```python
from build123d import *

# Parameters (mm, degrees)
ESQUISSE1_W             = 9.73
ESQUISSE1_H             = 5.03
BOSS_EXTRU_1_DEPTH      = 3.31
ESQUISSE3_W             = 3.841312789
ESQUISSE3_H             = 3.396529204
BOSS_EXTRU_2_DEPTH      = 0.1
BOSS_EXTRU_2_DEPTH_BACK = 1
ENL_V_MAT_EXTRU_1_DEPTH = 10.98001124
ESQUISSE5_W             = 5.874071128
ESQUISSE5_H             = 5.928896842
ENL_V_MAT_EXTRU_2_DEPTH = 2.1
ENL_V_MAT_EXTRU_4_DEPTH = 2.1
CONG_1_R                = 0.75
CONG_2_R                = 0.75


with BuildPart() as part:
    # Esquisse1 → Boss.-Extru.1 (new body)
    with BuildSketch(Plane.XY):
        Rectangle(ESQUISSE1_W, ESQUISSE1_H)
    extrude(amount=BOSS_EXTRU_1_DEPTH)

    # Esquisse3 → Boss.-Extru.2 (add, two sides)
    with BuildSketch(Plane(origin=(0, 0, 0), x_dir=(-1, 0, 0), z_dir=(0, 0, -1))) as boss_extru_2_sk:
        with Locations((-3.194354846, 0)):
            Rectangle(ESQUISSE3_W, ESQUISSE3_H)
        with Locations((3.194354846, 0)):
            Rectangle(ESQUISSE3_W, ESQUISSE3_H)
    extrude(amount=BOSS_EXTRU_2_DEPTH)
    extrude(boss_extru_2_sk.sketch, amount=-BOSS_EXTRU_2_DEPTH_BACK)

    # Esquisse4 → Enlèv. mat.-Extru.1 (cut, through all)
    with BuildSketch(Plane(origin=(4.865, 0, 0), x_dir=(0, 0, -1), z_dir=(1, 0, 0))):
        Polygon((-1.655, -2.515), (-3.31, -2.017151535), (-3.31, 2.017151535), (-1.655, 2.515), (-1.655, 2.602439027), (-3.426184741, 2.639019495), (-3.454926537, -2.688664416), (-1.655, -2.688664416), align=None)
    extrude(amount=-ENL_V_MAT_EXTRU_1_DEPTH, mode=Mode.SUBTRACT)

    # Esquisse5 → Enlèv. mat.-Extru.2 (cut)
    with BuildSketch(Plane.XY.offset(3.31)):
        with Locations((0, 0.049057066)):
            Rectangle(ESQUISSE5_W, ESQUISSE5_H)
    extrude(amount=-ENL_V_MAT_EXTRU_2_DEPTH, mode=Mode.SUBTRACT)

    # Esquisse6 → Enlèv. mat.-Extru.4 (cut)
    with BuildSketch(Plane.XY.offset(3.31)):
        Polygon((-2.937035564, 1.938709767), (-2.937035564, -1.938709767), (4.353991242, -1.938709767), (4.353991242, -0.833970123), (3.541647976, -0.833970123), (3.541647976, 0.833970123), (4.353991242, 0.833970123), (4.353991242, 1.938709767), align=None)
        Polygon((-4.353991242, -0.833970123), (-4.353991242, -1.938709767), (-2.937035564, -1.938709767), (-2.937035564, 1.938709767), (-4.353991242, 1.938709767), (-4.353991242, 0.833970123), (-3.541647976, 0.833970123), (-3.541647976, -0.833970123), align=None)
    extrude(amount=-ENL_V_MAT_EXTRU_4_DEPTH, mode=Mode.SUBTRACT)

    # Congé1
    cong_1_edges = [part.edges().sort_by_distance(p)[0] for p in [
        (-2.937035564, 2.226854883, 1.21),
        (2.937035564, 2.226854883, 1.21),
        (2.937035564, -2.226854883, 1.21),
        (-2.937035564, -2.226854883, 1.21),
    ]]
    fillet(cong_1_edges, radius=CONG_1_R)

    # Congé2
    cong_2_edges = [part.edges().sort_by_distance(p)[0] for p in [
        (2.937035564, 1.977930651, 3.31),
        (-2.937035564, -1.977930651, 3.31),
        (-2.937035564, 1.977930651, 3.31),
        (2.937035564, -1.977930651, 3.31),
    ]]
    fillet(cong_2_edges, radius=CONG_2_R)


solid = part.part
```
Geometry: final body of the model. Coordinates: model frame, mm. A direction names the side the tool comes from. Round coordinates to 2 decimals unless told otherwise and drop trailing zeros. Order: outer loops, then holes, each group sorted by start corner. A loop starts at its lowest first (then second) coordinate and runs counter-clockwise, first axis right, second up. Notation, with made-up numbers: (-2, -26) -> (8, -26) arc R10 cw to (8, -9) -> close; hole circle Ø11 at (3, 50). An arc over 180 degrees is marked (long way). Use CSV: the item, a comma, the result in double quotes. Start each with the question number.
1) Section D-D (z = 0.65). Return the cut outline in (x, y) (3 decimals), and give its area (3 significant figures).
2) First-contact query: pin 1 Ø1.5 at (x, z) = (4, 3) entering from +Y; pin 2 Ø3 at (x, y) = (-1.5, 0) entering from +Z; pin 3 Ø0.8 at (y, z) = (0, 2.5) entering from +X (3 decimals). Flat tips, straight axial feed; report the tip coordinate or a pass-through.
3) Set-up query: faces 1 (the face through (4, -0.834, 2)), 2 (the face through (3, 0, -0.1)). Return all of +Z, -Z, +X, -X, +Y, -Y with unobstructed straight access to the full face (end or side cutting, diameter ignored); none if empty.
4) Section A-A (z = 2.8). Return the cut outline in (x, y) (3 decimals), and give its area (3 significant figures).
5) Section C-C (y = -1.8). Return the cut outline in (x, z) (3 decimals), and give its area (3 significant figures).
6) Draft query along X for faces 3 (the face through (3.542, 0, 2)), 4 (the face through (5.115, 0, 0.4)), 5 (the face through (0, -2.515, 1)). Return one class per face: +X half, -X half, draft (parallel to the pull), parting line (faces both ways), or undercut.
7) Material intervals for line 1 along X through (y, z) = (-1.4, 2.55) (3 decimals); line 2 along X through (y, z) = (0.8, 3) (3 decimals); line 3 along Y through (x, z) = (4, 2.3), sorted ascending. Write a range as from..to.
8) Section B-B (x = 1.5). Return the cut outline in (y, z) (3 decimals).
Returned:
1,outline,"(-5.115, -1.698) -> (-4.865, -1.698) -> (-4.865, -2.515) -> (4.865, -2.515) -> (4.865, -1.698) -> (5.115, -1.698) -> (5.115, 1.698) -> (4.865, 1.698) -> (4.865, 2.515) -> (-4.865, 2.515) -> (-4.865, 1.698) -> (-5.115, 1.698) -> close"
1,area,"50.6 mm²"
2,pin 1,"stops at y = 2.34"
2,pin 2,"stops at z = 1.21"
2,pin 3,"stops at x = 4.865"
3,face 1,"+Z"
3,face 2,"-Z, +X, -X, +Y, -Y"
4,outline,"(-4.865, -2.171) -> (-2.976, -2.171) -> (-2.976, -1.939) -> (-4.354, -1.939) -> (-4.354, -0.834) -> (-3.542, -0.834) -> (-3.542, 0.834) -> (-4.354, 0.834) -> (-4.354, 1.939) -> (-2.976, 1.939) -> (-2.976, 2.171) -> (-4.865, 2.171) -> close; (2.976, -2.171) -> (4.865, -2.171) -> (4.865, 2.171) -> (2.976, 2.171) -> (2.976, 1.939) -> (4.354, 1.939) -> (4.354, 0.834) -> (3.542, 0.834) -> (3.542, -0.834) -> (4.354, -0.834) -> (4.354, -1.939) -> (2.976, -1.939) -> close"
4,area,"8.42 mm²"
5,outline,"(-4.865, 0) -> (4.865, 0) -> (4.865, 3.31) -> (4.354, 3.31) -> (4.354, 1.21) -> (-4.354, 1.21) -> (-4.354, 3.31) -> (-4.865, 3.31) -> close"
5,area,"13.9 mm²"
6,face 3,"undercut"
6,face 4,"+X half"
6,face 5,"draft"
7,line 1,"x = -4.865..-4.354, 4.354..4.865"
7,line 2,"x = -4.865..-3.542, 3.542..4.865"
7,line 3,"y = -2.32..-1.94, -0.83..0.83, 1.94..2.32"
8,outline,"(-2.515, 0) -> (-1.698, 0) -> (-1.698, -0.1) -> (1.698, -0.1) -> (1.698, 0) -> (2.515, 0) -> (2.515, 1.21) -> (-2.515, 1.21) -> close"
